Here's how the part is built. I have some questions about the finished solid (model axes, mm). Face numbers are marked on the shaded views. A direction names the side the tool comes from. Round coordinates to 2 decimals unless told otherwise and drop trailing zeros. Order: outer loops, then holes, each group sorted by start corner. A loop starts at its lowest first (then second) coordinate and runs counter-clockwise, first axis right, second up. Notation, with made-up numbers: (-33.5, 66) -> (25.5, 66) arc R27 ccw to (25.5, 100) -> close; hole circle Ø5 at (14.25, 24.5). An arc over 180 degrees is marked (long way). Use a Markdown table: item, result. Add a question column.
(1) I want a section at D-D, the plane z = 7. Please give me the cut outline in (x, y).
(2) If I drill on probe 1 along Z at (x, y) = (-9.5, -2.89); probe 2 along X at (y, z) = (-6.5, 8) (3 decimals); probe 3 along X at (y, z) = (-7, 11), over which ranges is the centre line in solid material (lowest first)?
(3) I want a section at A-A, the plane x = -3. Please give me the cut outline in (y, z) (3 decimals), then the cut area to 3 significant figures.
(4) On a 3-axis mill with a long thin cutter (end or side, diameter ignored), from which of +Z, -Z, +X, -X, +Y, -Y can I reach the whole of each face in a straight line? I mean the marked faces 1 and 2. Say none if no direction works.
(5) Thinking about a two-plate mould opening in Z: for the marked faces 3, 4, 5 and 6, which applies, pulls with the +Z half, pulls with the -Z half, needs draft (parallel to the pull), parting line crosses it, or undercut?
(6) I want a section at B-B, the plane z = 19. Please give me the cut outline in (x, y).
(7) I'm going to push flat-ended pins straight in: P1, Ø1.9, axis at y = 16, z = 33.5, coming from the -X side; P2, Ø2, axis at x = 3, z = 30, coming from the -Y side; P3, Ø10, axis at x = -5, z = 23.5, coming from the +Y side. Where does each tip first touch, or does it pass through?
from build123d import *

# Parameters (mm, degrees)
SKETCH1_W                         = 32
SKETCH1_H                         = 29
BOSS_EXTRUDE1_DEPTH               = 35
FILLET1_R                         = 2
SLOT_FOR_COIL_DEPTH               = 1
SLOT_FOR_COIL_DEPTH_BACK          = 30
BOSS_EXTRUDE2_DEPTH               = 7
BOSS_EXTRUDE3_DEPTH               = 1.75
SKETCH5_W                         = 2
SKETCH5_H                         = 7
SLOT_TO_FEED_IN_WIRE_DEPTH        = 33
SLOT_FO_PCB_DEPTH                 = 22
SKETCH7_W                         = 2
SKETCH7_H                         = 33
BOSS_EXTRUDE4_DEPTH               = 0.25
FILLET2_R                         = 6
ROD_MOUNT_SLOT_REACH              = 34
SKETCH14_W                        = 2.5
SKETCH14_H                        = 20
SIDE_CAVITY_FOR_MOUNT_PLATE_DEPTH = 22
SKETCH16_W                        = 2
SKETCH16_H                        = 2
SIDE_STOPS_FOR_MOUNT_PLATE_DEPTH  = 22
BOSS_EXTRUDE6_DEPTH               = 22
SKETCH21_W                        = 12
SKETCH21_H                        = 2
BOSS_EXTRUDE7_DEPTH               = 4
SKETCH23_W                        = 8
SKETCH23_H                        = 1.75
CUT_EXTRUDE7_DEPTH                = 2
FILLET3_R                         = 1
CUT_EXTRUDE8_REACH                = 34
SKETCH26_R                        = 5.25


with BuildPart() as part:
    # Sketch1 → Boss-Extrude1 (new body)
    with BuildSketch(Plane.XY):
        Rectangle(SKETCH1_W, SKETCH1_H)
    extrude(amount=BOSS_EXTRUDE1_DEPTH)

    # Fillet1
    fillet1_edges = [part.edges().sort_by_distance(p)[0] for p in [
        (16, -14.5, 17.5),
        (-16, -14.5, 17.5),
        (-16, 14.5, 17.5),
        (16, 14.5, 17.5),
    ]]
    fillet(fillet1_edges, radius=FILLET1_R)

    # Sketch2 → Slot for Coil (cut, two sides)
    with BuildSketch(Plane.XZ.offset(14.5)) as slot_for_coil_sk:
        Polygon((-9.125, 0), (-9.125, 1.75), (-11.125, 1.75), (-11.125, 5), (11.125, 5), (11.125, 1.75), (9.125, 1.75), (9.125, 0), align=None)
    extrude(amount=SLOT_FOR_COIL_DEPTH, mode=Mode.SUBTRACT)
    extrude(slot_for_coil_sk.sketch, amount=-SLOT_FOR_COIL_DEPTH_BACK, mode=Mode.SUBTRACT)

    # Sketch3 → Boss-Extrude2 (add)
    with BuildSketch(Plane.XZ.offset(14.5)):
        Polygon((-9.125, 0), (-9.125, 1.75), (-11.125, 1.75), (-11.125, 5), (11.125, 5), (11.125, 1.75), (9.125, 1.75), (9.125, 0), align=None)
    extrude(amount=-BOSS_EXTRUDE2_DEPTH)

    # Sketch4 → Boss-Extrude3 (add)
    with BuildSketch(Plane(origin=(0, 0, 1.75), x_dir=(-1, 0, 0), z_dir=(0, 0, -1))):
        with BuildLine():
            Line((-9.125, 7.5), (-9.125, 6.5))
            ThreePointArc((-9.125, 6.5), (-8.875, 7), (-9.125, 7.5))
        make_face()
    boss_extrude3 = extrude(amount=BOSS_EXTRUDE3_DEPTH)

    # Mirror1: Boss-Extrude3 across plane
    add(boss_extrude3.mirror(Plane(origin=(0, 0, 0), x_dir=(0, 0, 1), z_dir=(1, 0, 0))))

    # Sketch5 → slot to feed in wire (cut)
    with BuildSketch(Plane(origin=(0, 0, 0), x_dir=(-1, 0, 0), z_dir=(0, 0, -1))):
        with Locations((0, -11)):
            Rectangle(SKETCH5_W, SKETCH5_H)
    extrude(amount=-SLOT_TO_FEED_IN_WIRE_DEPTH, mode=Mode.SUBTRACT)

    # Sketch6 → slot fo PCB (cut)
    with BuildSketch(Plane(origin=(0, 14.5, 0), x_dir=(1, 0, 0), z_dir=(0, 1, 0))):
        Polygon((11.5, -7.5), (-11.5, -7.5), (-11.5, -29.5), (-12.5, -29.5), (-12.5, -33), (12.5, -33), (12.5, -29.5), (11.5, -29.5), align=None)
    extrude(amount=-SLOT_FO_PCB_DEPTH, mode=Mode.SUBTRACT)

    # Sketch7 → Boss-Extrude4 (add)
    with BuildSketch(Plane.XZ.offset(14.5)):
        with Locations((0, 16.5)):
            Rectangle(SKETCH7_W, SKETCH7_H)
    extrude(amount=-BOSS_EXTRUDE4_DEPTH)

    # Fillet2
    fillet2_edges = [part.edges().sort_by_distance(p)[0] for p in [
        (0, -14.25, 33),
    ]]
    fillet(fillet2_edges, radius=FILLET2_R)

    # Sketch11 → Rod Mount Slot (cut, up to next)
    with BuildSketch(Plane(origin=(16, 0, 44), x_dir=(0, 0, -1), z_dir=(1, 0, 0)), mode=Mode.PRIVATE) as rod_mount_slot_sk1:
        with BuildLine():
            Line((32.5, 25), (32.5, 0))
            ThreePointArc((32.5, 0), (26.5, -6), (20.5, 0))
            Line((20.5, 0), (20.5, 25))
            ThreePointArc((20.5, 25), (26.5, 31), (32.5, 25))
        make_face()
    rod_mount_slot_tool1 = extrude(rod_mount_slot_sk1.sketch, amount=-ROD_MOUNT_SLOT_REACH, mode=Mode.PRIVATE) & part.part
    add(rod_mount_slot_tool1.solids().sort_by_distance((16, 12.5, 17.5))[0], mode=Mode.SUBTRACT)

    # Sketch14 → Side cavity for mount plate (cut)
    with BuildSketch(Plane(origin=(0, 14.5, 0), x_dir=(1, 0, 0), z_dir=(0, 1, 0))):
        with Locations((12.75, -17.5)):
            Rectangle(SKETCH14_W, SKETCH14_H)
    extrude(amount=-SIDE_CAVITY_FOR_MOUNT_PLATE_DEPTH, mode=Mode.SUBTRACT)

    # Sketch16 → Side stops for mount plate (add)
    with BuildSketch(Plane(origin=(0, 14.5, 0), x_dir=(1, 0, 0), z_dir=(0, 1, 0))):
        with Locations((11, -8.5)):
            Rectangle(SKETCH16_W, SKETCH16_H)
        with Locations((11, -26.5)):
            Rectangle(SKETCH16_W, SKETCH16_H)
    extrude(amount=-SIDE_STOPS_FOR_MOUNT_PLATE_DEPTH)

    # Sketch20 → Boss-Extrude6 (add)
    with BuildSketch(Plane(origin=(0, 14.5, 0), x_dir=(1, 0, 0), z_dir=(0, 1, 0))):
        Polygon((11.5, -29.5), (10, -27.5), (11.5, -27.5), align=None)
        Polygon((10, -9.5), (8.5, -7.5), (10, -7.5), align=None)
    extrude(amount=-BOSS_EXTRUDE6_DEPTH)

    # Sketch21 → Boss-Extrude7 (add)
    with BuildSketch(Plane(origin=(0, 14.5, 0), x_dir=(-1, 0, 0), z_dir=(0, 1, 0))):
        with Locations((0, 34)):
            Rectangle(SKETCH21_W, SKETCH21_H)
    boss_extrude7 = extrude(amount=BOSS_EXTRUDE7_DEPTH)

    # Sketch23 → Cut-Extrude7 (cut)
    with BuildSketch(Plane.XY.offset(35)):
        with Locations((0, 15.875)):
            Rectangle(SKETCH23_W, SKETCH23_H)
    cut_extrude7 = extrude(amount=-CUT_EXTRUDE7_DEPTH, mode=Mode.SUBTRACT)

    # Mirror3: Boss-Extrude7, Cut-Extrude7 across plane
    add(boss_extrude7.mirror(Plane.ZX))
    add(cut_extrude7.mirror(Plane.ZX), mode=Mode.SUBTRACT)

    # Fillet3
    fillet3_edges = [part.edges().sort_by_distance(p)[0] for p in [
        (6, 14.5, 34),
        (-6, 14.5, 34),
        (6, 18.5, 34),
        (-6, 18.5, 34),
        (6, -18.5, 34),
        (-6, -18.5, 34),
        (6, -14.5, 34),
        (-6, -14.5, 34),
    ]]
    fillet(fillet3_edges, radius=FILLET3_R)

    # Sketch26 → Cut-Extrude8 (cut, up to next)
    with BuildSketch(Plane(origin=(-16, 0, 0), x_dir=(0, 0, -1), z_dir=(1, 0, 0)), mode=Mode.PRIVATE) as cut_extrude8_sk1:
        with Locations((-23.015, -2.89)):
            Circle(SKETCH26_R)
    cut_extrude8_tool1 = extrude(cut_extrude8_sk1.sketch, amount=CUT_EXTRUDE8_REACH, mode=Mode.PRIVATE) & part.part
    add(cut_extrude8_tool1.solids().sort_by_distance((-16, -2.89, 23.015))[0], mode=Mode.SUBTRACT)


solid = part.part
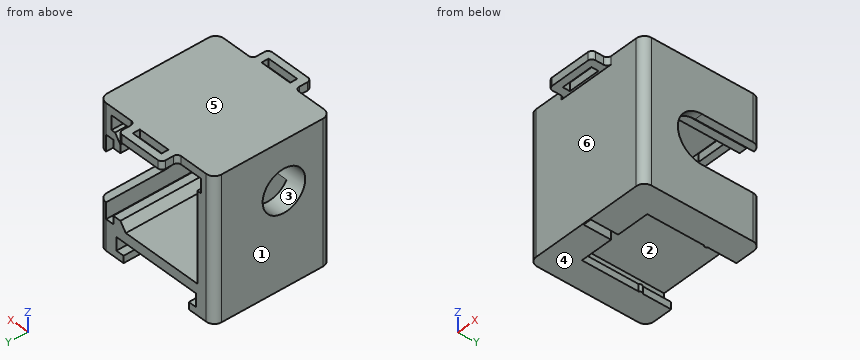
Taken from the geometry:
| question | item | result |
|---|---|---|
| 1 | outline | (-16, -12.5) arc R2 ccw to (-14, -14.5) -> (14, -14.5) arc R2 ccw to (16, -12.5) -> (16, 12.5) arc R2 ccw to (14, 14.5) -> (-14, 14.5) arc R2 ccw to (-16, 12.5) -> close; hole (-1, -14.25) -> (1, -14.25) -> (1, -7.5) -> (-1, -7.5) -> close |
| 2 | probe 1 | z = 0 to 1.75, 5 to 7.5, 33 to 35 |
| 2 | probe 2 | x = -16 to -11.5, 8.875 to 12, 14 to 16 |
| 2 | probe 3 | x = -16 to -11.5, 14 to 16 |
| 3 | outline | (-18.5, 33) -> (-16.75, 33) -> (-16.75, 35) -> (-18.5, 35) -> close; (-15, 33) -> (-14.5, 33) -> (-14.5, 0) -> (-7.5, 0) -> (-7.5, 5) -> (14.5, 5) -> (14.5, 7.5) -> (-7.5, 7.5) -> (-7.5, 20.503) arc R5.25 cw to (-7.5, 25.527) -> (-7.5, 33) -> (15, 33) -> (15, 35) -> (-15, 35) -> close; (16.75, 33) -> (18.5, 33) -> (18.5, 35) -> (16.75, 35) -> close |
| 3 | area | 351 mm2 |
| 4 | face 1 | +Z, -Z, -X, +Y, -Y |
| 4 | face 2 | +Y |
| 5 | face 3 | undercut |
| 5 | face 4 | pulls with the -Z half |
| 5 | face 5 | pulls with the +Z half |
| 5 | face 6 | needs draft |
| 6 | outline | (-16, -12.5) arc R2 ccw to (-14, -14.5) -> (14, -14.5) arc R2 ccw to (16, -12.5) -> (16, -5.81) -> (14, -5.81) -> (14, -7.5) -> (1, -7.5) -> (1, -14.25) -> (-1, -14.25) -> (-1, -7.5) -> (-11.5, -7.5) -> (-11.5, -6.27) -> (-16, -6.27) -> close; (-16, 0.49) -> (-11.5, 0.49) -> (-11.5, 14.5) -> (-14, 14.5) arc R2 ccw to (-16, 12.5) -> close |
| 7 | P1 | stops at x = -6.11 |
| 7 | P2 | stops at y = -14.5 |
| 7 | P3 | stops at y = -7.5 |
